Geometry check sheet. Reference: the model listing, model coordinates, mm. Round coordinates to 2 decimals unless told otherwise and drop trailing zeros. Order: outer loops, then holes, each group sorted by start corner. A loop starts at its lowest first (then second) coordinate and runs counter-clockwise, first axis right, second up.
Autodesk Inventor part; units mm, degrees
ref_plane "YZ Plane" through (0, 0, 0) normal (1, 0, 0) x (0, 1, 0)
ref_plane "XZ Plane" through (0, 0, 0) normal (0, 1, 0) x (-1, 0, 0)
ref_plane "XY Plane" through (0, 0, 0) normal (0, 0, 1) x (1, 0, 0)
sketch "Esboço1" plane through (0, 0, 0) normal (1, 0, 0) x (0, 1, 0)
  line L0 (1012, 0) -> (1012, -66)
  line L1 (0, -66) -> (0, 0)
  line L2 (1012, 0) -> (946, 0)
  line L3 (946, 0) -> (946, 6)
  line L4 (946, 6) -> (886, 6)
  line L5 (886, 6) -> (886, 0)
  line L6 (0, 0) -> (66, 0)
  line L7 (66, 0) -> (66, 6)
  line L8 (66, 6) -> (126, 6)
  line L9 (126, 6) -> (126, 0)
  line L10 (126, 0) -> (886, 0)
  line L11 (1012, -66) -> (942, -66)
  line L12 (942, -66) -> (942, -60)
  line L13 (942, -60) -> (882, -60)
  line L14 (882, -60) -> (882, -66)
  line L15 (0, -66) -> (66, -66)
  line L16 (66, -66) -> (66, -60)
  line L17 (66, -60) -> (126, -60)
  line L18 (126, -60) -> (126, -66)
  line L19 (126, -66) -> (882, -66)
  dimension "d0" = 1012
  dimension "d1" = 66
  dimension "d4" = 66
  dimension "d5" = 6
  dimension "d6" = 60
  dimension "d7" = 66
  dimension "d8" = 6
  dimension "d9" = 60
  dimension "d10" = 6
  dimension "d11" = 60
  dimension "d12" = 6
  dimension "d13" = 6
  dimension "d16" = 66
  dimension "d17" = 66
extrude "Extrusão1" add sketch "Esboço1" along normal blind 4
sketch "Esboço2" plane through (4, 0, 0) normal (1, 0, 0) x (0, 0, -1)
  point P0 (0, 0)
sketch "Esboço3" plane through (4, 0, 0) normal (1, 0, 0) x (0, 0, -1)
  point P0 (0, 0)
properties part number "PAREDES LAT-CONTRA"
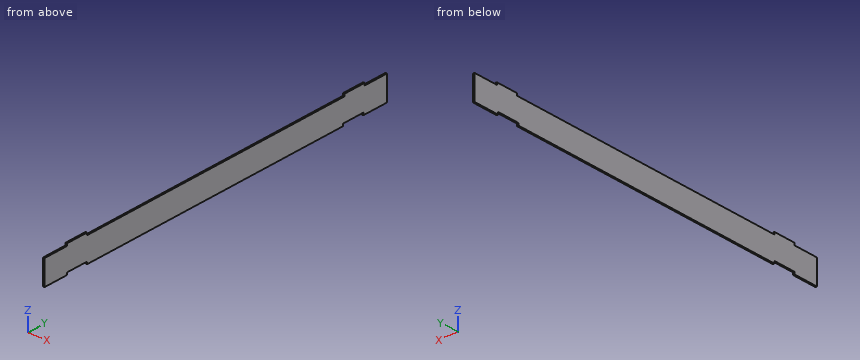
(1) Material ranges on line 1 (Y direction, x = 2.9, z = 2.5); line 2 (Z direction, x = 3.65, y = 684), recorded low to high.
Returned:
line 1: y = 66 to 126, 886 to 946
line 2: z = -66 to 0
(2) Sectioned sample at A-A, the plane x = 0.6. Record the cut outline in (y, z), and give its area (3 significant figures).
Returned:
outline: (0, -66) - (66, -66) - (66, -60) - (126, -60) - (126, -66) - (882, -66) - (882, -60) - (942, -60) - (942, -66) - (1012, -66) - (1012, 0) - (946, 0) - (946, 6) - (886, 6) - (886, 0) - (126, 0) - (126, 6) - (66, 6) - (66, 0) - (0, 0) - close
area: 66,800 mm2
(3) Sectioned sample at B-B, the plane y = 421.5. Record the cut outline in (x, z), and give its area (3 significant figures).
Returned:
outline: (0, -66) - (4, -66) - (4, 0) - (0, 0) - close
area: 264 mm2
(4) Depth check by flat-ended pin: P1, Ø2, axis at x = 2.5, z = 3.5, coming from the +Y side; P2, Ø2, axis at x = 3, z = 4, coming from the -Y side; P3, Ø2, axis at x = 3, y = 900.5, coming from the -Z side. Enter the tip coordinate at first touch or a pass-through.
Returned:
P1: stops at y = 946
P2: stops at y = 66
P3: stops at z = -60
